from build123d import *

# Parameters (mm, degrees)
BASES_W             = 12
BASES_H             = 12
BASE_DEPTH          = 0.2
EDGE_FLANGE1_DEPTH  = 12
EDGE_FLANGE2_DEPTH  = 12
EDGE_FLANGE3_DEPTH  = 12
EDGE_FLANGE4_DEPTH  = 12
VENTS_W             = 1.4
VENTS_H             = 0.8
VENT_DEPTH          = 10.052071586
VCP_COUNT           = 2
VCP_ANGLE           = 90
VCP_COPY_1_SKETCH_W = 1.4
VCP_COPY_1_SKETCH_H = 0.8
VCP_COPY_1_DEPTH    = 10.052071586


# Sheet-metal steps are written as plain solids
with BuildPart() as part:
    # BaseS → Base (new body)
    with BuildSketch(Plane(origin=(0, 1.6, 0), x_dir=(1, 0, 0), z_dir=(0, 1, 0))):
        Rectangle(BASES_W, BASES_H)
    extrude(amount=-BASE_DEPTH)

    # Edge-Flange1 section (across the edge) → Edge-Flange1 (add)
    with BuildSketch(Plane(origin=(6, 1.4, 6.1), x_dir=(0, 0, -1), z_dir=(-1, 0, 0))):
        with BuildLine():
            Line((-0.2, 0.1), (-0.2, 1.4))
            Line((-0.2, 1.4), (0, 1.4))
            Line((0, 1.4), (0, 0.1))
            ThreePointArc((0, 0.1), (0.029289322, 0.029289322), (0.1, 0))
            Line((0.1, 0), (0.1, -0.2))
            ThreePointArc((0.1, -0.2), (-0.112132034, -0.112132034), (-0.2, 0.1))
        make_face()
    extrude(amount=EDGE_FLANGE1_DEPTH)

    # Edge-Flange2 section (across the edge) → Edge-Flange2 (add)
    with BuildSketch(Plane(origin=(-6, 1.4, -6.1), x_dir=(0, 0, 1), z_dir=(1, 0, 0))):
        with BuildLine():
            Line((-0.2, 0.1), (-0.2, 1.4))
            Line((-0.2, 1.4), (0, 1.4))
            Line((0, 1.4), (0, 0.1))
            ThreePointArc((0, 0.1), (0.029289322, 0.029289322), (0.1, 0))
            Line((0.1, 0), (0.1, -0.2))
            ThreePointArc((0.1, -0.2), (-0.112132034, -0.112132034), (-0.2, 0.1))
        make_face()
    extrude(amount=EDGE_FLANGE2_DEPTH)

    # Edge-Flange3 section (across the edge) → Edge-Flange3 (add)
    with BuildSketch(Plane(origin=(6.1, 1.4, -6), x_dir=(-1, 0, 0), z_dir=(0, 0, 1))):
        with BuildLine():
            Line((-0.2, 0.1), (-0.2, 1.4))
            Line((-0.2, 1.4), (0, 1.4))
            Line((0, 1.4), (0, 0.1))
            ThreePointArc((0, 0.1), (0.029289322, 0.029289322), (0.1, 0))
            Line((0.1, 0), (0.1, -0.2))
            ThreePointArc((0.1, -0.2), (-0.112132034, -0.112132034), (-0.2, 0.1))
        make_face()
    extrude(amount=EDGE_FLANGE3_DEPTH)

    # Edge-Flange4 section (across the edge) → Edge-Flange4 (add)
    with BuildSketch(Plane(origin=(-6.1, 1.4, 6), x_dir=(1, 0, 0), z_dir=(0, 0, -1))):
        with BuildLine():
            Line((-0.2, 0.1), (-0.2, 1.4))
            Line((-0.2, 1.4), (0, 1.4))
            Line((0, 1.4), (0, 0.1))
            ThreePointArc((0, 0.1), (0.029289322, 0.029289322), (0.1, 0))
            Line((0.1, 0), (0.1, -0.2))
            ThreePointArc((0.1, -0.2), (-0.112132034, -0.112132034), (-0.2, 0.1))
        make_face()
    extrude(amount=EDGE_FLANGE4_DEPTH)

    # VentS → Vent (cut, symmetric)
    with BuildSketch(Plane(origin=(0, 0, 0), x_dir=(0, 0, -1), z_dir=(1, 0, 0))):
        with Locations((4.8, 0.4)):
            Rectangle(VENTS_W, VENTS_H)
    vent = extrude(amount=VENT_DEPTH, both=True, mode=Mode.SUBTRACT)

    # VHM: Vent across plane
    add(vent.mirror(Plane.XY), mode=Mode.SUBTRACT)

    # VCP: Vent ×2 about axis
    vcp_axis = Axis((0, 1.68, 0), (0, -1, 0))
    for i in range(1, VCP_COUNT):
        add(vent.rotate(vcp_axis, i * VCP_ANGLE / (VCP_COUNT - 1)), mode=Mode.SUBTRACT)

    # VCP copy 1 sketch → VCP copy 1 (cut, symmetric)
    with BuildSketch(Plane(origin=(0, 0, 0), x_dir=(-1, 0, 0), z_dir=(0, 0, 1))):
        with Locations((4.8, -0.4)):
            Rectangle(VCP_COPY_1_SKETCH_W, VCP_COPY_1_SKETCH_H)
    extrude(amount=VCP_COPY_1_DEPTH, both=True, mode=Mode.SUBTRACT)


solid = part.part
Check sheet for the modelled part. Datum: model origin and axes. Units: mm. A direction names the side the tool comes from. Coordinates: 2 decimals unless noted, no trailing zeros. Write each loop counter-clockwise with the first axis right and the second up, starting at its lowest first coordinate (ties: lowest second). Pieces come first, ordered by that corner, then holes.
Item 1: Cross-section at A-A on z = -0.75. Record the boundary of the cut face in (x, y), then the cut area to 3 significant figures.
Numbers:
outline: (-6.3, 0) - (-6.1, 0) - (-6.1, 1.3) arc R0.1 cw to (-6, 1.4) - (6, 1.4) arc R0.1 cw to (6.1, 1.3) - (6.1, 0) - (6.3, 0) - (6.3, 1.3) arc R0.3 ccw to (6, 1.6) - (-6, 1.6) arc R0.3 ccw to (-6.3, 1.3) - close
area: 3.05 mm2
Item 2: Scan lines: probe 1 along X at (y, z) = (1.2, -4.5); probe 2 along Y at (x, z) = (2.5, 3.75). Record each from-to range of solid material in increasing order.
Numbers:
probe 1: x = -6.3 to -6.1, 6.1 to 6.3
probe 2: y = 1.4 to 1.6
Item 3: Mould release check, pull along Z, two halves, no side actions. Record for faces 6 (the face through (0, 1, -6.3)), 7 (the face through (0, 1, 6.1)), 8 (the face through (6.1, 1, 0)): released by +Z, released by -Z, zero draft, split by the parting line, or undercut.
Numbers:
face 6: released by -Z
face 7: undercut
face 8: zero draft
Item 4: Access from +Z, -Z, +X, -X, +Y, -Y to the whole of each face (thin tool, end or side, straight path). Record for faces 1 (the face through (0, 1.6, 0)), 2 (the face through (6.3, 1, 0)), 3 (the face through (-6.1, 1, 0)), 4 (the face through (0, 1, -6.1)), 5 (the face through (0, 1.4, 0)).
Numbers:
face 1: +Z, -Z, +X, -X, +Y
face 2: +Z, -Z, +X, +Y, -Y
face 3: +Z, -Z, -Y
face 4: +X, -X, -Y
face 5: -Y
Item 5: Cross-section at B-B on x = 3. Record the boundary of the cut face in (y, z), then the cut area to 3 significant figures.
Numbers:
outline: (0, -6.3) - (1.3, -6.3) arc R0.3 ccw to (1.6, -6) - (1.6, 6) arc R0.3 ccw to (1.3, 6.3) - (0, 6.3) - (0, 6.1) - (1.3, 6.1) arc R0.1 cw to (1.4, 6) - (1.4, -6) arc R0.1 cw to (1.3, -6.1) - (0, -6.1) - close
area: 3.05 mm2
Item 6: Cross-section at C-C on y = 0.4. Count the separate pieces of the cut face and the enclosed holes in it, then the cut area to 3 significant figures.
Numbers:
separate pieces: 12
enclosed holes: 0
area: 7.36 mm2
